Work out the finished part from the listing and answer in its coordinate system (mm). Give positions to 0.01 mm unless a question says otherwise; leave off trailing zeros. Loops run counter-clockwise (first coordinate to the right, second up) from the corner with the lowest first, then second, coordinate; pieces in that order, holes last. Notation, with made-up numbers: M -6,-9 L 37,-9 A13 cw 37,3 Z; hole C 32.25,70 d11. An arc over 180 degrees is marked long. Write item = value, one per line. Start each with the question number.
1. Flat-ended cylindrical pins translate along their axes: pin 1 Ø1 at (y, z) = (10.5, 10) entering from -X; pin 2 Ø3 at (y, z) = (3.5, 9.5) entering from +X; pin 3 Ø1.5 at (x, z) = (-18, 10.5) entering from -Y; pin 4 Ø4 at (x, y) = (-43.5, 3) entering from -Z. Find the tip coordinate at first contact, or state that the pin passes through.
2. Consider L1, parallel to X at y = 7.5, z = 0.75; L2, parallel to X at y = -2.5, z = 5.25; L3, parallel to Y at x = 0, z = 3.5. Determine where each line is inside the solid, lowest interval first. Write a range as [from, to].
3. Section D-D on x = 58 is taken. Determine the outline of the cut face in (y, z), plus the area to 3 significant figures.
4. The mould has two halves that part along X. Classify faces 1 (the face through (-3.279, -14.768, 6.261)), 2 (the face through (-57.1, -11.4, 6.3)): released by +X, released by -X, zero draft, split by the parting line, or undercut.
5. Section B-B on x = 0 is taken. Determine the outline of the cut face in (y, z), plus the area to 3 significant figures.
6. Section A-A on z = 9.75 is taken. Determine the outline of the cut face in (x, y), plus the area to 3 significant figures.
7. Section C-C on y = 0 is taken. Determine the outline of the cut face in (x, z), plus the area to 3 significant figures.
```python
from build123d import *

# Parameters (mm, degrees)
F0_R     = 11.687263
F0_R_2   = 15.127238
F1_DEPTH = 12.7


with BuildPart() as f1:
    # F0 (on Top) → F1 (new body)
    with BuildSketch(Plane.XY):
        with BuildLine():
            Line((52.713767, 17.888913), (54.524425, 17.888913))
            ThreePointArc((54.524425, 17.888913), (72.413338, 0), (54.524425, -17.888913))
            Line((54.524425, -17.888913), (52.713767, -17.888913))
            ThreePointArc((52.713767, -17.888913), (72.504739, 0), (52.713767, 17.888913))
        make_face()
        with BuildLine():
            Line((-54.524425, 17.888913), (-52.831878, 17.888913))
            ThreePointArc((-52.831878, 17.888913), (-72.49323, 0), (-52.831878, -17.888913))
            Line((-52.831878, -17.888913), (-54.524425, -17.888913))
            ThreePointArc((-54.524425, -17.888913), (-72.413338, 0), (-54.524425, 17.888913))
        make_face()
        with BuildLine():
            ThreePointArc((54.524425, -17.888913), (72.413338, 0), (54.524425, 17.888913))
            Line((54.524425, 17.888913), (52.713767, 17.888913))
            Line((52.713767, 17.888913), (-52.831878, 17.888913))
            Line((-52.831878, 17.888913), (-54.524425, 17.888913))
            ThreePointArc((-54.524425, 17.888913), (-72.413338, 0), (-54.524425, -17.888913))
            Line((-54.524425, -17.888913), (-52.831878, -17.888913))
            Line((-52.831878, -17.888913), (52.713767, -17.888913))
            Line((52.713767, -17.888913), (54.524425, -17.888913))
        make_face()
        with Locations((-54.524425, 0)):
            Circle(F0_R, mode=Mode.SUBTRACT)
        Circle(F0_R_2, mode=Mode.SUBTRACT)
        with Locations((54.524425, 0)):
            Circle(F0_R, mode=Mode.SUBTRACT)
    extrude(amount=F1_DEPTH)


solid = f1.part
```
Verdict:
q1.pin_1 = -69.45
q1.pin_2 = 72.39
q1.pin_3 = -17.89
q1.pin_4 = 0
q2.L1 = [-70.85, -63.49], [-45.56, -13.14], [13.14, 45.56], [63.49, 70.87]
q2.L2 = [-72.32, -65.94], [-43.11, -14.92], [14.92, 43.11], [65.94, 72.33]
q2.L3 = [-17.89, -15.13], [15.13, 17.89]
q3.outline = M -17.64,0 L -11.16,0 L -11.16,12.7 L -17.64,12.7 Z; M 11.16,0 L 17.64,0 L 17.64,12.7 L 11.16,12.7 Z
q3.area = 165 mm2
q4.face_1 = undercut
q4.face_2 = undercut
q5.outline = M -17.89,0 L -15.13,0 L -15.13,12.7 L -17.89,12.7 Z; M 15.13,0 L 17.89,0 L 17.89,12.7 L 15.13,12.7 Z
q5.area = 70.1 mm2
q6.outline = M -52.83,-17.89 L 52.71,-17.89 A17.98 ccw long 52.71,17.89 L -52.83,17.89 A17.97 ccw long Z; hole C -54.52,0 d23.37; hole C 0,0 d30.25; hole C 54.52,0 d23.37
q6.area = 3,340 mm2
q7.outline = M -72.49,0 L -66.21,0 L -66.21,12.7 L -72.49,12.7 Z; M -42.84,0 L -15.13,0 L -15.13,12.7 L -42.84,12.7 Z; M 15.13,0 L 42.84,0 L 42.84,12.7 L 15.13,12.7 Z; M 66.21,0 L 72.5,0 L 72.5,12.7 L 66.21,12.7 Z
q7.area = 864 mm2
